For this review, take the finished solid that the model builds, in its own axes (mm). Coordinates: 2 decimals unless noted, no trailing zeros. Write each loop counter-clockwise with the first axis right and the second up, starting at its lowest first coordinate (ties: lowest second). Pieces come first, ordered by that corner, then holes.
```python
from build123d import *

# Parameters (mm, degrees)
F0_W     = 58
F0_H     = 124
F0_R     = 11
F1_DEPTH = 1
F2_R     = 10
F3_R     = 0.6


with BuildPart() as f1:
    # F0 (on Top) → F1 (new body)
    with BuildSketch(Plane.XY):
        Rectangle(F0_W, F0_H)
        with BuildLine():
            ThreePointArc((-20, 49.5), (-25, 54.5), (-20, 59.5))
            Line((-20, 59.5), (-10, 59.5))
            ThreePointArc((-10, 59.5), (-5, 54.5), (-10, 49.5))
            Line((-10, 49.5), (-20, 49.5))
        make_face(mode=Mode.SUBTRACT)
        Circle(F0_R, mode=Mode.SUBTRACT)
    extrude(amount=F1_DEPTH)

    # F2
    f2_edges = [f1.edges().sort_by_distance(p)[0] for p in [
        (-29, -62, 0.5),
        (29, -62, 0.5),
        (29, 62, 0.5),
        (-29, 62, 0.5),
    ]]
    fillet(f2_edges, radius=F2_R)

    # F3
    f3_edges = [f1.edges().sort_by_distance(p)[0] for p in [
        (29, 0, 1),
        (26.071068, -59.071068, 1),
        (26.071068, 59.071068, 1),
        (0, -62, 1),
        (0, 62, 1),
        (-26.071068, -59.071068, 1),
        (-26.071068, 59.071068, 1),
        (-29, 0, 1),
        (-25, 54.5, 1),
        (-15, 59.5, 1),
        (-5, 54.5, 1),
        (-15, 49.5, 1),
        (-11, 0, 1),
    ]]
    fillet(f3_edges, radius=F3_R)


solid = f1.part
```
Q1. For probe 1 along Y at (x, z) = (0, 0.3); probe 2 along Y at (x, z) = (-5.5, 0.1); probe 3 along X at (y, z) = (-1.5, 0.35), list the stretches that pass through material, from the lowest coordinate up.
Ans:
probe 1: y = -62 to -11, 11 to 62
probe 2: y = -62 to -9.53, 9.53 to 52.32, 56.68 to 62
probe 3: x = -29 to -10.9, 10.9 to 29
Q2. Clearance check with a flat-ended pin moving along its axis: pin 1 Ø13 at (x, y) = (0, 0) entering from -Z. State where the tip first meets the part, or that it passes through.
Ans:
pin 1: passes through
Q3. Draft analysis for pull direction X (two halves, no side actions). For faces 1 (the cylindrical face through (-5, 54.6, 0.2)), 2 (the cylindrical face through (-25, 54.4, 0.2)), 3 (the flat face through (0, -13, 1)), 4 (the cylindrical face through (-26.15, 58.99, 0.2)), state which applies: +X half, -X half, draft (parallel to the pull), parting line (faces both ways), or undercut.
Ans:
face 1: undercut
face 2: undercut
face 3: draft
face 4: -X half
Q4. Add section A-A (x = 0). State the section outline as (y, z) points.
Ans:
outline: (-62, 0) - (-11, 0) - (-11, 0.4) arc R0.6 ccw to (-11.6, 1) - (-61.4, 1) arc R0.6 ccw to (-62, 0.4) - close; (11, 0) - (62, 0) - (62, 0.4) arc R0.6 ccw to (61.4, 1) - (11.6, 1) arc R0.6 ccw to (11, 0.4) - close
Q5. Add section C-C (z = 0.25). State the section outline as (x, y) points, then the cut area to 3 significant figures.
Ans:
outline: (-29, -52) arc R10 ccw to (-19, -62) - (19, -62) arc R10 ccw to (29, -52) - (29, 52) arc R10 ccw to (19, 62) - (-19, 62) arc R10 ccw to (-29, 52) - close; hole (-20, 49.5) - (-10, 49.5) arc R5 ccw to (-10, 59.5) - (-20, 59.5) arc R5 ccw to start; hole circle Ø22 at (0, 0)
area: 6,550 mm2
Q6. Add section D-D (x = -8). Give the number of separate pieces and of enclosed holes in the cut face, then the cut area to 3 significant figures.
Ans:
separate pieces: 3
enclosed holes: 0
area: 99.2 mm2
Q7. Add section B-B (y = 0). State the section outline as (x, z) points, then the cut area to 3 significant figures.
Ans:
outline: (-29, 0) - (-11, 0) - (-11, 0.4) arc R0.6 ccw to (-11.6, 1) - (-28.4, 1) arc R0.6 ccw to (-29, 0.4) - close; (11, 0) - (29, 0) - (29, 0.4) arc R0.6 ccw to (28.4, 1) - (11.6, 1) arc R0.6 ccw to (11, 0.4) - close
area: 35.7 mm2
